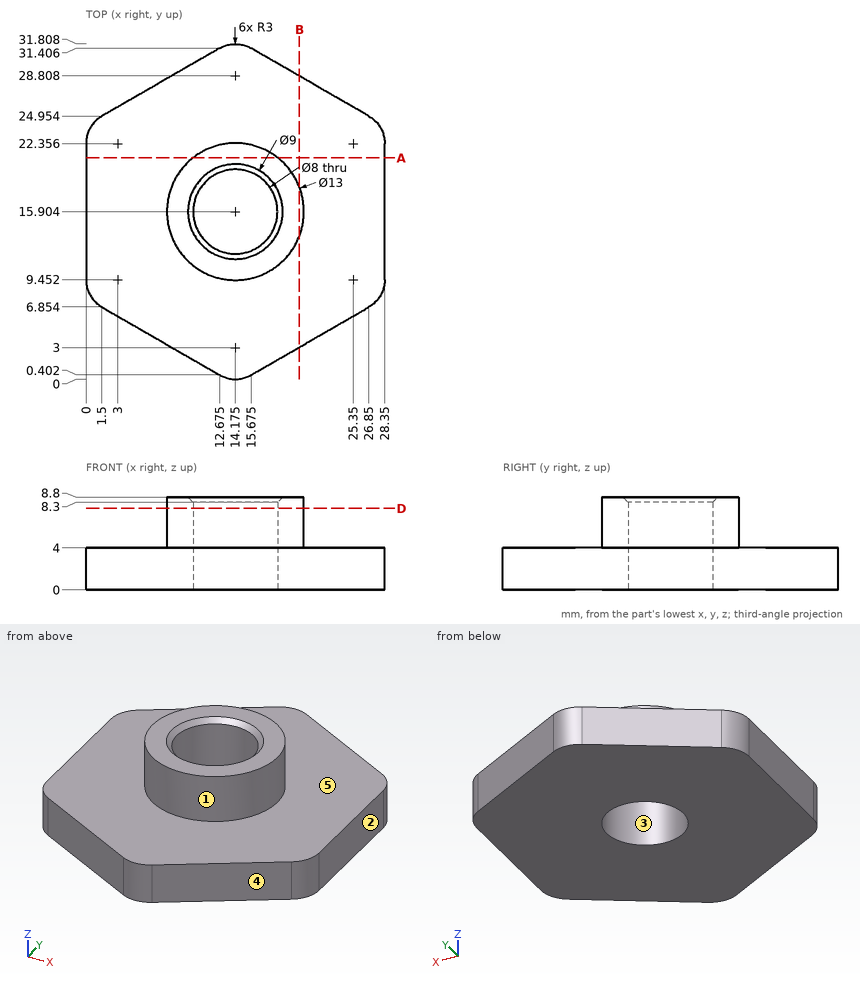
Geometry check sheet. Reference: drawing and pictorial views, mm from the part's lowest x, y, z. A direction names the side the tool comes from. Round coordinates to 2 decimals unless told otherwise and drop trailing zeros. Order: outer loops, then holes, each group sorted by start corner. A loop starts at its lowest first (then second) coordinate and runs counter-clockwise, first axis right, second up. Notation, with made-up numbers: (55.5, 40.5) - (98.5, 40.5) arc R29 cw to (98.5, 74.5) - close; hole circle Ø11 at (-19.75, 47). An arc over 180 degrees is marked (long way). Use a Markdown table: item, result. Add a question column.
1) Section check B-B (x = 20.25). Record the cut outline in (y, z) (1 decimal).
2) Section check A-A (y = 21). Record the cut outline in (x, z), then the cut area to 3 significant figures.
3) Set-up check for the marked faces 1 and 2: record each of +Z, -Z, +X, -X, +Y, -Y from which the full face is reachable in a straight line by a thin tool's end or side.
4) Mould release check, pull along Y, two halves, no side actions. Record for the marked faces 3, 4 and 5: released by +Y, released by -Y, zero draft, split by the parting line, or undercut.
5) Thickness scan on line 1 along Z through (x, y) = (7.75, 22.5); line 2 along X through (y, z) = (18.5, 7) (1 decimal); line 3 along X through (y, z) = (13, 7.75) (1 decimal). Record the ranges inside material, lowest first.
6) Gauge pin test, flat ends, axial feed: P1, Ø1, axis at y = 10.5, z = 5, coming from the -X side; P2, Ø4, axis at y = 25.5, z = 4, coming from the -X side; P3, Ø5, axis at x = 14.18, y = 15.9, coming from the +Z side. Record the tip position at first contact, or that the pin passes through.
7) Section check D-D (z = 7.75). Record the cut outline in (x, y) (1 decimal).
Established:
| question | item | result |
|---|---|---|
| 1 | outline | (3, 0) - (28.8, 0) - (28.8, 4) - (18.2, 4) - (18.2, 8.8) - (13.6, 8.8) - (13.6, 4) - (3, 4) - close |
| 2 | outline | (0, 0) - (28.35, 0) - (28.35, 4) - (18.21, 4) - (18.21, 8.8) - (10.14, 8.8) - (10.14, 4) - (0, 4) - close |
| 2 | area | 152 mm2 |
| 3 | face 1 | +Z |
| 3 | face 2 | +Z, -Z, +X, +Y, -Y |
| 4 | face 3 | undercut |
| 4 | face 4 | released by -Y |
| 4 | face 5 | zero draft |
| 5 | line 1 | 0 to 4 |
| 5 | line 2 | 8.2 to 11.1, 17.2 to 20.1 |
| 5 | line 3 | 8.4 to 11.4, 16.9 to 20 |
| 6 | P1 | x = 9.91 |
| 6 | P2 | x = 0.23 |
| 6 | P3 | through |
| 7 | outline | circle Ø13 at (14.2, 15.9); hole circle Ø8 at (14.2, 15.9) |
